Autodesk Inventor part; units mm, degrees
ref_plane "РабПлоскость1" through (1, 0, 0) normal (1, 0, 0) x (0, 1, 0)
ref_plane "РабПлоскость2" through (-1, 0, 0) normal (1, 0, 0) x (0, 1, 0)
ref_plane "XZ Plane" through (0, 0, 0) normal (0, 1, 0) x (-1, 0, 0)
sketch "Эскиз1" plane through (0, 0, 0) normal (0, 0, 1) x (1, 0, 0)
  circle A0 centre (0, 0) radius 3
  dimension "d0" = 6
extrude "Выдавливание1" add sketch "Эскиз1" along normal blind 20
fillet "Сопряжение1" radius 0.5 2 edges at (-3, 0, 20) (-3, 0, 0)
sketch "Эскиз2" plane through (0, 0, 0) normal (0, 0, -1) x (-1, 0, 0)
  circle A0 centre (0, 0) radius 2.25
  circle A1 centre (1, 0) radius 0.5
  circle A2 centre (-1, 0) radius 0.5
  line L0 (0, 2.25) -> (0, -2.5)
  circle A3 centre (0, 0) radius 2.5
  dimension "d4" = 4.5
  dimension "d5" = 1
  dimension "d6" = 1
  dimension "d7" = 2
extrude "Выдавливание2" cut sketch "Эскиз2" against normal blind 1 contours A0 L0 | L0 A0
ref_plane "РабПлоскость1" through (1, 0, 0) normal (1, 0, 0) x (0, 1, 0)
sketch "Эскиз3" plane through (1, 0, 0) normal (1, 0, 0) x (0, 1, 0)
  line L0 (0, 0) -> (0, -2)
  arc A0 (0, -2) -> (5.0002, -6.9531) centre (4.9534, -2) ccw
  line L1 (5.0002, -6.9531) -> (10.0002, -6.9531)
  dimension "d11" = 2
  dimension "d12" = 5
sketch "Эскиз4" plane through (1, 0, 0) normal (0, 0, -1) x (-1, 0, 0)
  circle A0 centre (0, 0) radius 0.5
  circle A1 centre (2, 0) radius 0.5
  circle A2 centre (2, 0) radius 0.5
  point P0 (1, 0)
sweep "Сдвиг1" add profiles "Эскиз4" path "Эскиз3" contours A0
ref_plane "РабПлоскость2" through (-1, 0, 0) normal (1, 0, 0) x (0, 1, 0)
sketch "Эскиз5" plane through (-1, 0, 0) normal (1, 0, 0) x (0, 1, 0)
  line L0 (0, 0) -> (0, -2)
  line L1 (-0.5, -2) -> (0.5, -2)
  line L2 (5.005, -7.4531) -> (4.9955, -6.4532)
  arc A0 (0, -2) -> (5.0002, -6.9531) centre (4.9076, -2.0462) ccw
  line L3 (5.0002, -6.9531) -> (10.0002, -6.9531)
  line L4 (10.0002, -7.4531) -> (10.0002, -6.4531)
sweep "Сдвиг2" add profiles "Эскиз4" path "Эскиз5" path curves L0 A0 L3 contours A1
properties part number "heater-cartrig" material "Messing, weicher Gelbton"
Design review of the part built by this model. Coordinates are the model's own, in mm. A direction names the side the tool comes from. Give positions to 0.01 mm unless a question says otherwise; leave off trailing zeros. Order: outer loops, then holes, each group sorted by start corner. A loop starts at its lowest first (then second) coordinate and runs counter-clockwise, first axis right, second up. Notation, with made-up numbers: (79.25, 66) - (133.25, 66) arc R13 ccw to (133.25, 90) - close; hole circle Ø2 at (50, 74). An arc over 180 degrees is marked (long way). Use a Markdown table: item, result. Add a question column.
(1) Machinability: for faces 1 (the face through (1.4, -0.3, -0.5)), 2 (the face through (-3, 0, 10)), which of the approach directions +Z, -Z, +X, -X, +Y, -Y give a long, thin tool a straight path to every point of the face, cutting with its end or side? Answer none if there is none.
(2) Add section C-C on y = 1.75. Give the number of separate pieces and of enclosed holes in the cut face, then the cut area to 3 significant figures.
(3) Add section B-B on z = 8.75. Give the boundary of the cut face in (x, y), then the cut area to 3 significant figures.
(4) Wall thickness on probe 1 along Y at (x, z) = (0, 0.65); probe 2 along X at (y, z) = (0.25, -3); probe 3 along Y at (x, z) = (0.2, 9.5): over which ranges is each line inside the solid? List them lowest first. Write a range as [from, to].
(5) Clearance check with a flat-ended pin moving along its axis: P1, Ø1.1, axis at x = -1, z = -7, coming from the +Y side. State where the tip first meets the part, or that it passes through.
(6) Add section A-A on x = 0. Give the boundary of the cut face in (y, z).
(7) Mouldability with a two-part tool opening along Z and no side actions: class faces 3 (the face through (0, 0, 20)), 4 (the face through (-1, 10, -7)), 5 (the face through (-0.93, 7.53, -6.46)), 6 (the face through (0, 0, 1)) as +Z half, -Z half, draft (parallel to the pull), parting line (faces both ways), or undercut.
Report:
| question | item | result |
|---|---|---|
| 1 | face 1 | none |
| 1 | face 2 | +Z |
| 2 | separate pieces | 3 |
| 2 | enclosed holes | 0 |
| 2 | area | 96.4 mm² |
| 3 | outline | circle Ø6 at (0, 0) |
| 3 | area | 28.3 mm² |
| 4 | probe 1 | y = [-3, -2.25], [2.25, 3] |
| 4 | probe 2 | x = [-1.48, -0.52], [0.52, 1.48] |
| 4 | probe 3 | y = [-2.99, 2.99] |
| 5 | P1 | stops at y = 10 |
| 6 | outline | (-3, 0.5) arc R0.5 ccw to (-2.5, 0) - (-2.25, 0) - (-2.25, 1) - (2.25, 1) - (2.25, 0) - (2.5, 0) arc R0.5 ccw to (3, 0.5) - (3, 19.5) arc R0.5 ccw to (2.5, 20) - (-2.5, 20) arc R0.5 ccw to (-3, 19.5) - close |
| 7 | face 3 | +Z half |
| 7 | face 4 | draft |
| 7 | face 5 | parting line |
| 7 | face 6 | undercut |
